Part model, mm, in its own coordinate system. A direction names the side the tool comes from. Give positions to 0.01 mm unless a question says otherwise; leave off trailing zeros. Write each loop counter-clockwise with the first axis right and the second up, starting at its lowest first coordinate (ties: lowest second). Pieces come first, ordered by that corner, then holes. Notation, with made-up numbers: M 18.5,55 L 37.5,55 A22 cw 37.5,92 Z; hole C -5.75,-16.5 d6. An arc over 180 degrees is marked long. Answer as CSV lines item,"result". Start each with the question number.
1) Slice it at C-C, the plane y = 67. Give the cut face in (x, z).
2) Wall check: line 1 along Z through (x, y) = (-87, -142); line 2 along X through (y, z) = (-123, 1.5); line 3 along Z through (x, y) = (52.5, 29). Give the ranges that are in metal, low to high. Write a range as from..to.
3) Mould opens along Y. For faces 5 (the cylindrical face through (-85.687, -130.28, 17.844)), 6 (the flat face through (-75, -150, 15)), 7 (the cylindrical face through (75.4, 44.9, 14.9)) say: pulls with the +Y half, pulls with the -Y half, needs draft (parallel to the pull), parting line crosses it, or undercut.
4) Pin check, flat tips, straight feed: pin 1 Ø3.5 at (x, z) = (-87.5, 15) entering from -Y; pin 2 Ø1.5 at (x, z) = (23, 16.5) entering from -Y; pin 3 Ø8 at (x, z) = (-87.5, 15) entering from +Y. Stop position of each tip, or through.
5) Slice it at B-B, the plane y = -77.5. Give the cut face in (x, z), plus the area to 3 significant figures.
6) Slice it at A-A, the plane y = -113.5. Give the cut face in (x, z).
7) Slice it at D-D, the plane x = 87.5. Give the cut face in (y, z).
8) Tool access for faces 1 (the flat face through (75, -150, 15)), 2 (the flat face through (87, -110, 15)), 3 (the flat face through (50, -33, 8)), 4 (the flat face through (75, -26, 10.098)): list every direction of +Z, -Z, +X, -X, +Y, -Y with a clear straight run to the whole face (end or side of a thin tool).
```python
from build123d import *

# Parameters (mm, degrees)
F0_W     = 100
F0_H     = 50
F1_DEPTH = 30
F2_R     = 20
F3_R     = 3.37312
F4_DEPTH = 40
F6_DEPTH = 200.001


with BuildPart() as f1:
    # F0 (on Top) → F1 (new body)
    with BuildSketch(Plane.XY):
        with BuildLine():
            Line((-50, 100), (-50, 150))
            ThreePointArc((-50, 150), (-86.471849, 117.169906), (-100, 70))
            Line((-100, 70), (-100, -150))
            Line((-100, -150), (-50, -150))
            Line((-50, -150), (-50, 100))
        make_face()
        with Locations((0, 125)):
            Rectangle(F0_W, F0_H)
        with BuildLine():
            ThreePointArc((100, 70), (86.471849, 117.169906), (50, 150))
            Line((50, 150), (50, 100))
            Line((50, 100), (50, -150))
            Line((50, -150), (100, -150))
            Line((100, -150), (100, 70))
        make_face()
    extrude(amount=F1_DEPTH)

    # F2
    f2_edges = [f1.edges().sort_by_distance(p)[0] for p in [
        (-50, 100, 15),
        (50, 100, 15),
    ]]
    fillet(f2_edges, radius=F2_R)

    # F3 (on face) → F4 (cut)
    with BuildSketch(Plane.XZ.offset(150)):
        with Locations((-87.5, 15)):
            Circle(F3_R)
        with Locations((-62.5, 15)):
            Circle(F3_R)
        with Locations((62.5, 15)):
            Circle(F3_R)
        with Locations((87.5, 15)):
            Circle(F3_R)
    extrude(amount=-F4_DEPTH, mode=Mode.SUBTRACT)

    # F5 (on face) → F6 (cut, through all)
    with BuildSketch(Plane.YZ.offset(100)):
        with BuildLine():
            Line((-90, 10.0978), (40, 10.0978))
            ThreePointArc((40, 10.0978), (44.9022, 15), (40, 19.9022))
            Line((40, 19.9022), (-90, 19.9022))
            ThreePointArc((-90, 19.9022), (-94.9022, 15), (-90, 10.0978))
        make_face()
    extrude(amount=-F6_DEPTH, mode=Mode.SUBTRACT)


solid = f1.part
```
Found:
1,outline,"M -100,0 L -50,0 L -50,30 L -100,30 Z; M 50,0 L 100,0 L 100,30 L 50,30 Z"
2,line 1,"0..11.66, 18.34..30"
2,line 2,"-100..-50, 50..100"
2,line 3,"0..10.1, 19.9..30"
3,face 5,"needs draft"
3,face 6,"pulls with the -Y half"
3,face 7,"undercut"
4,pin 1,"y = -110"
4,pin 2,"y = 100"
4,pin 3,"y = 121.62"
5,outline,"M -100,0 L -50,0 L -50,10.1 L -100,10.1 Z; M -100,19.9 L -50,19.9 L -50,30 L -100,30 Z; M 50,0 L 100,0 L 100,10.1 L 50,10.1 Z; M 50,19.9 L 100,19.9 L 100,30 L 50,30 Z"
5,area,"2,020 mm²"
6,outline,"M -100,0 L -50,0 L -50,30 L -100,30 Z; M 50,0 L 100,0 L 100,30 L 50,30 Z; hole C -87.5,15 d6.75; hole C -62.5,15 d6.75; hole C 62.5,15 d6.75; hole C 87.5,15 d6.75"
7,outline,"M -150,0 L 115.48,0 L 115.48,30 L -150,30 L -150,18.37 L -110,18.37 L -110,11.63 L -150,11.63 Z; hole M -90,10.1 L 40,10.1 A4.9 ccw 40,19.9 L -90,19.9 A4.9 ccw Z"
8,face 1,"+Z, -Z, +X, -X, -Y"
8,face 2,"-Y"
8,face 3,"+Z, -Z, -Y"
8,face 4,"+X, -X"
